```python
from build123d import *

# Parameters (mm, degrees)
F0_W     = 101.6
F0_H     = 49.463168
F0_W_2   = 91.44
F0_H_2   = 39.303168
F1_DEPTH = 50.8
F2_R     = 5.08
F3_DEPTH = 114.3
F4_W     = 50.8
F4_H     = 22.569782
F5_DEPTH = 63.5


with BuildPart() as f1:
    # F0 (on Top) → F1 (new body)
    with BuildSketch(Plane.XY):
        with Locations((5.092576, 1.704902)):
            Rectangle(F0_W, F0_H)
        with Locations((5.092576, 1.704902)):
            Rectangle(F0_W_2, F0_H_2, mode=Mode.SUBTRACT)
    extrude(amount=F1_DEPTH)

    # F2 (on face) → F3 (cut)
    with BuildSketch(Plane.YZ.offset(55.892576)):
        with Locations((1.704902, 25.4)):
            Circle(F2_R)
    extrude(amount=-F3_DEPTH, mode=Mode.SUBTRACT)

    # F4 (on face) → F5 (cut)
    with BuildSketch(Plane.XZ.offset(23.026682)):
        with Locations((5.092576, 39.515109)):
            Rectangle(F4_W, F4_H)
    extrude(amount=-F5_DEPTH, mode=Mode.SUBTRACT)


solid = f1.part
```
CAD build for the part. Positions are in the model's coordinates, mm. A direction names the side the tool comes from. Give positions to 0.01 mm unless a question says otherwise; leave off trailing zeros. Loops run counter-clockwise (first coordinate to the right, second up) from the corner with the lowest first, then second, coordinate; pieces in that order, holes last. Notation, with made-up numbers: M 19.25,63 L 43.25,63 A12 ccw 43.25,84 Z; hole C -34,-32 d9. An arc over 180 degrees is marked long. Use one line per item in the form item = value.
Item 1: Slice it at A-A (x = -27). List the corners of the cut face in (y, z).
Determined:
outline = M -23.03,0 L -17.95,0 L -17.95,50.8 L -23.03,50.8 Z; M 21.36,0 L 26.44,0 L 26.44,50.8 L 21.36,50.8 Z
Item 2: Slice it at B-B (z = 25.4). List the corners of the cut face in (x, y), plus the area to 3 significant figures.
Determined:
outline = M -45.71,-23.03 L 55.89,-23.03 L 55.89,-3.38 L 50.81,-3.38 L 50.81,-17.95 L -40.63,-17.95 L -40.63,-3.38 L -45.71,-3.38 Z; M -45.71,6.78 L -40.63,6.78 L -40.63,21.36 L 50.81,21.36 L 50.81,6.78 L 55.89,6.78 L 55.89,26.44 L -45.71,26.44 Z
area = 1,330 mm2
Item 3: Flat gauge pins, fed straight in: pin 1 (5.5 mm diameter, centred on x = -7.5, y = 25, fed in from +Z); pin 2 (5 mm diameter, centred on x = 12.5, z = 31.5, fed in from +Y). Where does each tip first touch, or does it go through?
Determined:
pin_1 = 28.23
pin_2 = through
Item 4: Two-plate mould, pull along Y, no slides. Class faces 4 (the face through (4, 26.436, 19)), 5 (the face through (-45.707, 7, 25)), 6 (the face through (50.813, 1, 31)): pulls with the +Y half, pulls with the -Y half, needs draft (parallel to the pull), parting line crosses it, or undercut.
Determined:
face_4 = pulls with the +Y half
face_5 = needs draft
face_6 = undercut
Item 5: Slice it at D-D (z = 11.5). List the corners of the cut face in (x, y).
Determined:
outline = M -45.71,-23.03 L 55.89,-23.03 L 55.89,26.44 L -45.71,26.44 Z; hole M -40.63,-17.95 L 50.81,-17.95 L 50.81,21.36 L -40.63,21.36 Z
Item 6: Which spindle directions (+Z, -Z, +X, -X, +Y, -Y) get a long thin tool onto all of the face, cutting with end or side? Do faces 1 (the face through (-40.627, 1, 31)), 2 (the face through (30.493, -21, 39)), 3 (the face through (53.388, 1.044, 30.437)). Say none if no direction does.
Determined:
face_1 = +Z, -Z
face_2 = +Z, +Y, -Y
face_3 = +X, -X
Item 7: Drill centre lines: probe 1 along X at (y, z) = (15.5, 10); probe 2 along Y at (x, z) = (7, 18); probe 3 along X at (y, z) = (24.5, 40). Where is each one in solid material? Low to high. Write a range as from..to.
Determined:
probe_1 = -45.71..-40.63, 50.81..55.89
probe_2 = -23.03..-17.95, 21.36..26.44
probe_3 = -45.71..-20.31, 30.49..55.89
Item 8: Slice it at C-C (y = -19). List the corners of the cut face in (x, z), plus the area to 3 significant figures.
Determined:
outline = M -45.71,0 L 55.89,0 L 55.89,50.8 L 30.49,50.8 L 30.49,28.23 L -20.31,28.23 L -20.31,50.8 L -45.71,50.8 Z
area = 4,010 mm2
